```python
from build123d import *

# Parameters (mm, degrees)
SKETCH006_W      = 75
SKETCH006_H      = 80
EXTRUDE005_DEPTH = 2.5
EXTRUDE006_DEPTH = 2.5


with BuildPart() as extrude005:
    with BuildSketch(Plane.XY.offset(73)):
        Rectangle(SKETCH006_W, SKETCH006_H)
    extrude(amount=EXTRUDE005_DEPTH)


with BuildPart() as fusion:
    with BuildSketch(Plane.XY.offset(78)):
        with BuildLine():
            ThreePointArc((-34.5, 48), (-35.207107, 47.707107), (-35.5, 47))
            Line((-35.5, -47), (-35.5, 47))
            ThreePointArc((-35.5, -47), (-35.207107, -47.707107), (-34.5, -48))
            Line((34.5, -48), (-34.5, -48))
            ThreePointArc((34.5, -48), (35.207107, -47.707107), (35.5, -47))
            Line((35.5, 47), (35.5, -47))
            ThreePointArc((35.5, 47), (35.207107, 47.707107), (34.5, 48))
            Line((-34.5, 48), (34.5, 48))
        make_face()
    extrude(amount=-EXTRUDE006_DEPTH)

    # Fusion: union Extrude005
    add(extrude005.part)


solid = fusion.part
```
Can you work these out from the model? Positions are in its coordinate system, mm. A direction names the side the tool comes from. Coordinates: 2 decimals unless noted, no trailing zeros. Loops run counter-clockwise (first coordinate to the right, second up) from the corner with the lowest first, then second, coordinate; pieces in that order, holes last. Notation, with made-up numbers: M -15.5,13 L 11.5,13 A23 ccw 11.5,29 Z; hole C -29,58.5 d4. An arc over 180 degrees is marked long. Put each result on its own line as item: value. Start each with the question number.
(1) I need wall thicknesses on probe 1 along Y at (x, z) = (-10, 75.4); probe 2 along X at (y, z) = (5.5, 76.75); probe 3 along Z at (x, y) = (20, 41.5). Which ranges of each line are inside material? Lowest first, please.
(2) Which directions (+Z, -Z, +X, -X, +Y, -Y) give clear straight access to the entire face, cutting with the end or side of a thin tool? Please do faces 1 (the face through (-1, 40, 74)), 2 (the face through (35.5, 1, 77)), 3 (the face through (-35.5, -1, 77)), 4 (the face through (-1, -40, 74)).
(3) Imagine slicing it at B-B on z = 76.3. List the corners of the cut face in (x, y) for me, and give its area (3 significant figures).
(4) Imagine slicing it at C-C on y = 42.5. List the corners of the cut face in (x, z) for me.
(5) Imagine slicing it at A-A on x = 22. List the corners of the cut face in (y, z) for me.
(6) Will these pins go through, and if not, where does the flat tip stop? pin 1 Ø0.8 at (y, z) = (18, 76.5) entering from -X; pin 2 Ø1.2 at (x, z) = (-2.5, 73.5) entering from -Y; pin 3 Ø9 at (x, y) = (-1, -45.5) entering from -Z.
Worked answers:
1. probe 1: y = -40 to 40
1. probe 2: x = -35.5 to 35.5
1. probe 3: z = 75.5 to 78
2. face 1: -Z, +X, -X, +Y
2. face 2: +Z, +X, +Y, -Y
2. face 3: +Z, -X, +Y, -Y
2. face 4: -Z, +X, -X, -Y
3. outline: M -35.5,-47 A1 ccw -34.5,-48 L 34.5,-48 A1 ccw 35.5,-47 L 35.5,47 A1 ccw 34.5,48 L -34.5,48 A1 ccw -35.5,47 Z
3. area: 6,820 mm2
4. outline: M -35.5,75.5 L 35.5,75.5 L 35.5,78 L -35.5,78 Z
5. outline: M -48,75.5 L -40,75.5 L -40,73 L 40,73 L 40,75.5 L 48,75.5 L 48,78 L -48,78 Z
6. pin 1: stops at x = -35.5
6. pin 2: stops at y = -40
6. pin 3: stops at z = 75.5
